from build123d import *

# Parameters (mm, degrees)
F0_W     = 125
F0_H     = 100
F2_DEPTH = 63.5
F0_H_2   = 30
F3_DEPTH = 63.5
F1_R     = 37.5
F4_DEPTH = 2.5
F6_DEPTH = 5


with BuildPart() as f2:
    # F0 (on Front) → F2 (new body)
    with BuildSketch(Plane.XZ):
        with Locations((0, 17.5)):
            Rectangle(F0_W, F0_H)
    extrude(amount=-F2_DEPTH)

    # F0 (on Front) → F3 (join)
    with BuildSketch(Plane.XZ):
        with Locations((0, -47.5)):
            Rectangle(F0_W, F0_H_2)
    extrude(amount=-F3_DEPTH)

    # F1 (on Front) → F4 (cut, symmetric)
    with BuildSketch(Plane.XZ):
        with Locations((-13.5, 22.6666666667)):
            Circle(F1_R)
    extrude(amount=F4_DEPTH, both=True, mode=Mode.SUBTRACT)

    # F5 (on face) → F6 (cut)
    with BuildSketch(Plane.XY.offset(67.5)):
        Polygon((-57.5, 59), (-57.5, 50.3397459622), (-52.5, 59), align=None)
        Polygon((-57.5, 41.6794919243), (-57.5, 33.0192378865), (-42.5, 59), (-47.5, 59), align=None)
        Polygon((-57.5, 24.3589838486), (-57.5, 15.6987298108), (-32.5, 59), (-37.5, 59), align=None)
        Polygon((-27.5, 59), (-57.5, 7.0384757729), (-57.5, 5.5), (-53.3882394016, 5.5), (-22.5, 59), align=None)
        Polygon((-17.5, 59), (-48.3882394016, 5.5), (-43.3882394016, 5.5), (-12.5, 59), align=None)
        Polygon((-7.5, 59), (-38.3882394016, 5.5), (-33.3882394016, 5.5), (-2.5, 59), align=None)
        Polygon((2.5, 59), (-28.3882394016, 5.5), (-23.3882394016, 5.5), (7.5, 59), align=None)
        Polygon((-18.3882394016, 5.5), (-13.3882394016, 5.5), (17.5, 59), (12.5, 59), align=None)
        Polygon((-8.3882394016, 5.5), (-3.3882394016, 5.5), (27.5, 59), (22.5, 59), align=None)
        Polygon((1.6117605984, 5.5), (6.6117605984, 5.5), (37.5, 59), (32.5, 59), align=None)
        Polygon((11.6117605984, 5.5), (16.6117605984, 5.5), (47.5, 59), (42.5, 59), align=None)
        Polygon((21.6117605984, 5.5), (26.6117605984, 5.5), (57.5, 59), (52.5, 59), align=None)
        Polygon((31.6117605984, 5.5), (36.6117605984, 5.5), (57.5, 41.6794919243), (57.5, 50.3397459622), align=None)
        Polygon((41.6117605984, 5.5), (46.6117605984, 5.5), (57.5, 24.3589838486), (57.5, 33.0192378865), align=None)
        Polygon((51.6117605984, 5.5), (56.6117605984, 5.5), (57.5, 7.0384757729), (57.5, 15.6987298108), align=None)
    extrude(amount=-F6_DEPTH, mode=Mode.SUBTRACT)


solid = f2.part
Model file for the job. Use its own axes, mm. Give positions to 0.01 mm unless a question says otherwise; leave off trailing zeros. Loops run counter-clockwise (first coordinate to the right, second up) from the corner with the lowest first, then second, coordinate; pieces in that order, holes last. Notation, with made-up numbers: (38, 70) -> (48, 70) arc R23 ccw to (48, 79) -> close; hole circle Ø6 at (37, 71). An arc over 180 degrees is marked (long way). Use a Markdown table: item, result. Add a question column.
(1) Drop flat-ended pins along their axis: pin 1 Ø4 at (x, z) = (55, 65) entering from -Y; pin 2 Ø3 at (x, z) = (-36.5, 50) entering from -Y. Give the stop position or say it passes through.
(2) Wall check: line 1 along Z through (x, y) = (-13, 2); line 2 along Z through (x, y) = (24.5, 42); line 3 along Y through (x, z) = (-27, 41). Give the ranges that are in metal, low to high.
(3) Slice it at A-A on z = 33. List the corners of the cut face in (x, y), and give its area (3 significant figures).
(4) Mould opens along X. For faces 1 (the flat face through (-1, 24, 67.5)), 2 (the flat face through (-2.73, 32.62, 65.04)) say: +X half, -X half, draft (parallel to the pull), parting line (faces both ways), or undercut.
(5) Slice it at B-B on z = 14. List the corners of the cut face in (x, y).
Filled sheet:
| question | item | result |
|---|---|---|
| 1 | pin 1 | y = 0 |
| 1 | pin 2 | y = 2.5 |
| 2 | line 1 | -62.5 to -14.83, 60.16 to 67.5 |
| 2 | line 2 | -62.5 to 62.5 |
| 2 | line 3 | 2.5 to 63.5 |
| 3 | outline | (-62.5, 0) -> (-49.55, 0) -> (-49.55, 2.5) -> (22.55, 2.5) -> (22.55, 0) -> (62.5, 0) -> (62.5, 63.5) -> (-62.5, 63.5) -> close |
| 3 | area | 7,760 mm2 |
| 4 | face 1 | draft |
| 4 | face 2 | undercut |
| 5 | outline | (-62.5, 0) -> (-49.98, 0) -> (-49.98, 2.5) -> (22.98, 2.5) -> (22.98, 0) -> (62.5, 0) -> (62.5, 63.5) -> (-62.5, 63.5) -> close |
